Read the model definition and answer for the solid it produces. Units are mm, in the model's axes. A direction names the side the tool comes from. Coordinates: 2 decimals unless noted, no trailing zeros. Write each loop counter-clockwise with the first axis right and the second up, starting at its lowest first coordinate (ties: lowest second). Pieces come first, ordered by that corner, then holes.
Item 1: Each of these flat-tipped pins is pushed along its axis until it touches: P1, Ø5.5, axis at y = -27, z = 17, coming from the +X side; P2, Ø4, axis at x = -7.5, z = 14, coming from the -Y side; P3, Ø1, axis at x = -9, z = 4.5, coming from the -Y side. Where does it stop, or does it pass through?
Item 2: A tool of negligible diameter and unlimited length cuts with its end or side. For faces 4 (the face through (11, -16.175, 28)), 5 (the face through (-5, 11, 28)), 6 (the face through (-9, -22, 4)), from which of +Z, -Z, +X, -X, +Y, -Y can it reach the whole face along a straight path? Write none if from no direction.
Item 3: Section D-D (x = 0) is taken. Give the vertices of the cut face in (y, z) (3 decimals).
Item 4: Section C-C (z = 26) is taken. Give the vertices of the cut face in (x, y) (3 decimals).
Item 5: Straight lines are drawn through the part: probe 1 along Y at (x, z) = (0, 1.95) (3 decimals); probe 2 along Z at (x, y) = (19, -19); probe 3 along X at (y, z) = (-15.5, 26.5). For each, find the intervals that lie inside material, in ascending order.
Item 6: Determine the mould class of faces 1 (the face through (9, -11, 3)), 2 (the face through (-10, -25, 3)), 3 (the face through (0, -1, 0)) for opening direction Z: released by +Z, released by -Z, zero draft, split by the parting line, or undercut.
Item 7: Section A-A (y = -11.65) is taken. Give the vertices of the cut face in (x, z), then the cut area to 4 significant figures.
Item 8: Section B-B (x = -11.5) is taken. Give the vertices of the cut face in (y, z) (3 decimals).
from build123d import *

# Parameters (mm, degrees)
PAD_DEPTH       = 30
POCKET_DEPTH    = 20
POCKET001_DEPTH = 6.9
SKETCH004_R     = 9.5
POCKET002_DEPTH = 5
SKETCH005_W     = 10
SKETCH005_H     = 10
POCKET003_DEPTH = 5
SKETCH006_R     = 9.5
POCKET004_DEPTH = 56


with BuildPart() as part:
    # Sketch → Pad (new body)
    with BuildSketch(Plane.XY):
        Polygon((-21, 25.2), (-21, -28.9), (14, -28.9), (14, -22), (21, -22), (21, 25.2), align=None)
    extrude(amount=PAD_DEPTH)

    # Sketch001 → Pocket (cut)
    with BuildSketch(Plane.XY.offset(5)):
        Polygon((-15.5, 18.3), (-15.5, -22), (11.5, -22), (11.5, -28.9), (14, -28.9), (14, -22), (21, -22), (21, -18), (27.5, -18), (27.5, -12), (21, -12), (21, 12.2), (21, 12.2), (21, 18.2), (21, 18.2), (21, 25.2), (11.5, 25.2), (11.5, 18.3), align=None)
    extrude(amount=POCKET_DEPTH, mode=Mode.SUBTRACT)

    # Sketch003 → Pocket001 (cut)
    with BuildSketch(Plane(origin=(-15.5, -28.9, 3), x_dir=(1, 0, 0), z_dir=(0, -1, 0))):
        Polygon((20.030856, 9.535838), (10, 0), (0, 0), (0, 19.5), (20, 19.5), align=None)
    extrude(amount=-POCKET001_DEPTH, mode=Mode.SUBTRACT)

    # Sketch004 → Pocket002 (cut)
    with BuildSketch(Plane.XY.offset(5)):
        with Locations((0, 11.525)):
            Circle(SKETCH004_R)
        Polygon((-16, -5.475), (-16, -17), (9, -17), (9, -16.114332), (9, -5.475), align=None)
    extrude(amount=-POCKET002_DEPTH, mode=Mode.SUBTRACT)

    # Sketch005 → Pocket003 (cut)
    with BuildSketch(Plane.XY.offset(30)):
        Polygon((-16, -0.975), (-16, -22), (7, -22), (7, -16.175392), (16, -16.175392), (16, -0.975), align=None)
        with Locations((0, 11.525)):
            Rectangle(SKETCH005_W, SKETCH005_H)
    extrude(amount=-POCKET003_DEPTH, mode=Mode.SUBTRACT)

    # Sketch006 → Pocket004 (cut)
    with BuildSketch(Plane.YZ.offset(-22)):
        with Locations((-11.65, 15)):
            Circle(SKETCH006_R)
    extrude(amount=POCKET004_DEPTH, mode=Mode.SUBTRACT)


solid = part.part
Established:
1. P1: stops at x = 11.5
1. P2: stops at y = 18.3
1. P3: stops at y = -22
2. face 4: +Z
2. face 5: +Z, -Z
2. face 6: -Y
3. outline: (-28.9, 0) - (-17, 0) - (-17, 5) - (-22, 5) - (-22, 8.229) - (-28.9, 8.229) - close; (-28.9, 22.5) - (-22, 22.5) - (-22, 30) - (-28.9, 30) - close; (-5.475, 0) - (2.025, 0) - (2.025, 5) - (-5.475, 5) - close; (-0.975, 25) - (6.525, 25) - (6.525, 30) - (-0.975, 30) - close; (16.525, 25) - (18.3, 25) - (18.3, 5) - (21.025, 5) - (21.025, 0) - (25.2, 0) - (25.2, 30) - (16.525, 30) - close
4. outline: (-21, -28.9) - (14, -28.9) - (14, -22) - (21, -22) - (21, 25.2) - (-21, 25.2) - close; hole (-16, -22) - (7, -22) - (7, -16.175) - (16, -16.175) - (16, -0.975) - (-16, -0.975) - close; hole (-5, 6.525) - (5, 6.525) - (5, 16.525) - (-5, 16.525) - close
5. probe 1: y = -28.9 to -17, -5.475 to 2.025, 21.025 to 25.2
5. probe 2: z = 0 to 5, 25 to 30
5. probe 3: x = -21 to -16, 16 to 21
6. face 1: zero draft
6. face 2: undercut
6. face 3: released by -Z
7. outline: (-21, 0) - (-16, 0) - (-16, 5) - (-15.5, 5) - (-15.5, 5.5) - (-21, 5.5) - close; (-21, 24.5) - (-15.5, 24.5) - (-15.5, 25) - (-16, 25) - (-16, 30) - (-21, 30) - close; (9, 0) - (21, 0) - (21, 5) - (9, 5) - close; (16, 25) - (21, 25) - (21, 30) - (16, 30) - close
7. area: 140.5 mm2
8. outline: (-28.9, 0) - (-17, 0) - (-17, 5) - (-22, 5) - (-22, 3) - (-28.9, 3) - close; (-28.9, 22.5) - (-22, 22.5) - (-22, 30) - (-28.9, 30) - close; (-5.475, 0) - (25.2, 0) - (25.2, 30) - (-0.975, 30) - (-0.975, 25) - (18.3, 25) - (18.3, 5) - (-5.475, 5) - close
